Could you check a few things on this drawing? It's one solid part, dimensions in mm from its lowest x, y, z. A direction names the side the tool comes from. Give positions to 0.01 mm unless a question says otherwise; leave off trailing zeros. Write each loop counter-clockwise with the first axis right and the second up, starting at its lowest first coordinate (ties: lowest second). Pieces come first, ordered by that corner, then holes. Notation, with made-up numbers: (-29.75, -21) - (-6.75, -21) arc R24 ccw to (-6.75, -5) - close; hole circle Ø6 at (-36.5, 61.5). An arc over 180 degrees is marked (long way). One line per item, written item: value. Start each with the question number.
1) On a 3-axis mill with a long thin cutter (end or side, diameter ignored), from which of +Z, -Z, +X, -X, +Y, -Y can I reach the whole of each face in a straight line? I mean the marked faces 1 and 2. Say none if no direction works.
2) I'm going to push flat-ended pins straight in: P1, Ø3, axis at x = 12.5, y = 6, coming from the -Z side; P2, Ø5, axis at x = 6.5, z = 14.5, coming from the +Y side. Where does each tip first touch, or does it pass through?
3) Imagine slicing it at A-A on x = 16.51. Write out the boundary of the cut face in (y, z), plus the area to 3 significant figures.
4) Imagine slicing it at B-B on y = 0.5. Write out the boundary of the cut face in (x, z) (1 decimal).
5) Imagine slicing it at D-D on x = 26.5. Write out the boundary of the cut face in (y, z).
6) Imagine slicing it at C-C on z = 10. Write out the boundary of the cut face in (x, y).
7) Please list where these lines run through material, in increasing order: L1, parallel to X at y = 2.5, z = 16 (1 decimal); L2, parallel to Y at x = 14, z = 2; L3, parallel to X at y = 2, z = 7. Write a range as [from, to].
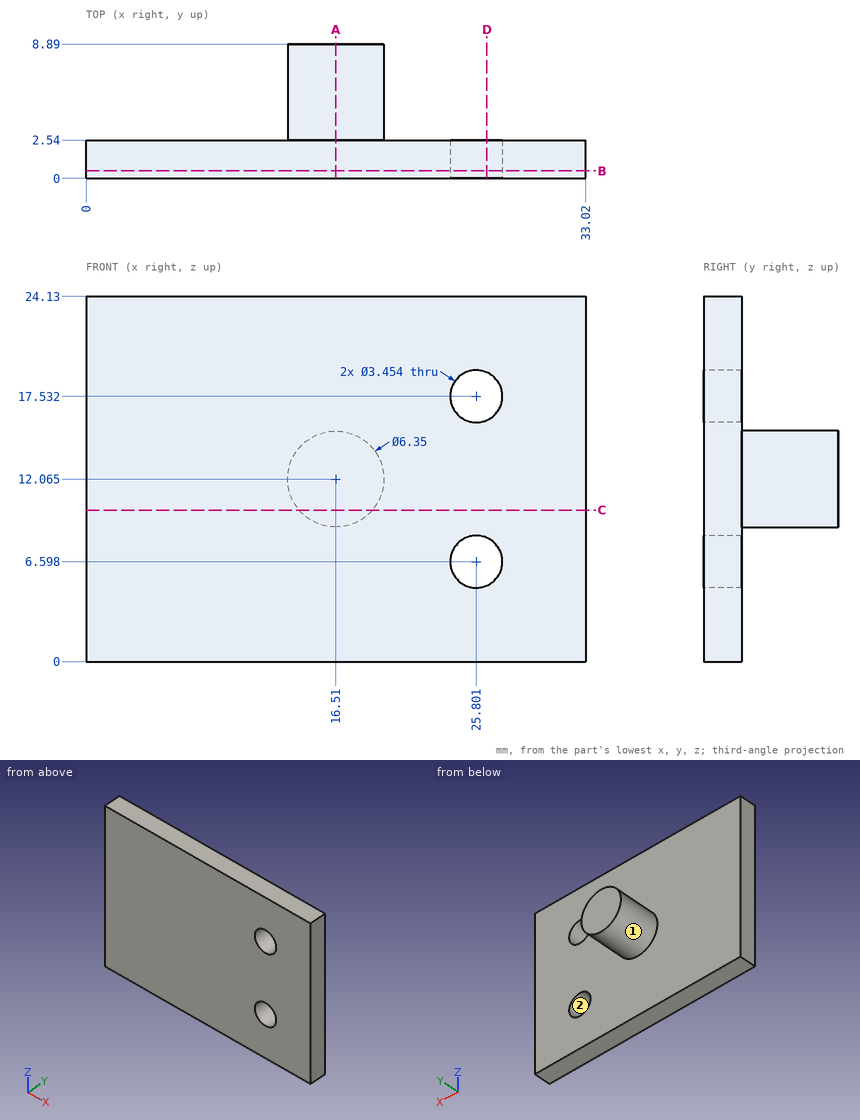
Numbers:
1. face 1: +Y
1. face 2: +Y, -Y
2. P1: z = 10.12
2. P2: y = 2.54
3. outline: (0, 0) - (2.54, 0) - (2.54, 8.89) - (8.89, 8.89) - (8.89, 15.24) - (2.54, 15.24) - (2.54, 24.13) - (0, 24.13) - close
3. area: 102 mm^2
4. outline: (0, 0) - (33, 0) - (33, 24.1) - (0, 24.1) - close; hole circle Ø3.5 at (25.8, 6.6); hole circle Ø3.5 at (25.8, 17.5)
5. outline: (0, 0) - (2.54, 0) - (2.54, 5.02) - (0, 5.02) - close; (0, 8.18) - (2.54, 8.18) - (2.54, 15.95) - (0, 15.95) - close; (0, 19.11) - (2.54, 19.11) - (2.54, 24.13) - (0, 24.13) - close
6. outline: (0, 0) - (33.02, 0) - (33.02, 2.54) - (18.92, 2.54) - (18.92, 8.89) - (14.1, 8.89) - (14.1, 2.54) - (0, 2.54) - close
7. L1: [0, 25], [26.6, 33]
7. L2: [0, 2.54]
7. L3: [0, 24.12], [27.48, 33.02]
